Autodesk Inventor part; units mm, degrees
ref_plane "YZ Plane" through (0, 0, 0) normal (1, 0, 0) x (0, 1, 0)
ref_plane "XZ Plane" through (0, 0, 0) normal (0, 1, 0) x (-1, 0, 0)
ref_plane "XY Plane" through (0, 0, 0) normal (0, 0, 1) x (1, 0, 0)
sketch "Sketch1" plane through (0, 0, 0) normal (1, 0, 0) x (0, 1, 0)
  line L0 (0, 0) -> (-127, 0)
  line L1 (-127, 0) -> (-127, -127)
  line L2 (-127, -127) -> (0, -127)
  line L3 (0, -127) -> (0, -120.65)
  line L4 (0, -6.35) -> (0, 0)
  line L5 (0, -6.35) -> (-3.175, -6.35)
  line L6 (-3.175, -6.35) -> (-3.175, -3.175)
  line L7 (-3.175, -3.175) -> (-9.525, -3.175)
  line L8 (-9.525, -3.175) -> (-9.525, -6.35)
  line L9 (-3.175, -6.35) -> (0, -6.35)
  line L10 (0, -120.65) -> (-3.175, -120.65)
  line L11 (-3.175, -120.65) -> (-3.175, -123.825)
  line L12 (-3.175, -123.825) -> (-9.525, -123.825)
  line L13 (-9.525, -123.825) -> (-9.525, -120.65)
  line L14 (0, -120.65) -> (-3.175, -120.65)
  line L15 (-120.65, -6.35) -> (-120.65, -9.525)
  line L16 (-120.65, -9.525) -> (-123.825, -9.525)
  line L17 (-123.825, -9.525) -> (-123.825, -15.875)
  line L18 (-123.825, -15.875) -> (-120.65, -15.875)
  line L19 (-120.65, -9.525) -> (-120.65, -6.35)
  line L20 (-120.65, -120.65) -> (-120.65, -117.475)
  line L21 (-120.65, -117.475) -> (-123.825, -117.475)
  line L22 (-123.825, -117.475) -> (-123.825, -111.125)
  line L23 (-123.825, -111.125) -> (-120.65, -111.125)
  line L24 (-120.65, -120.65) -> (-120.65, -117.475)
  line L25 (-120.65, -111.125) -> (-120.65, -15.875)
  line L26 (-120.65, -6.35) -> (-107.95, -6.35)
  line L27 (-107.95, -6.35) -> (-107.95, -3.175)
  line L28 (-107.95, -3.175) -> (-101.6, -3.175)
  line L29 (-101.6, -3.175) -> (-101.6, -6.35)
  line L30 (-120.65, -6.35) -> (-107.95, -6.35)
  line L31 (-101.6, -6.35) -> (-9.525, -6.35)
  line L32 (-120.65, -120.65) -> (-107.95, -120.65)
  line L33 (-107.95, -120.65) -> (-107.95, -123.825)
  line L34 (-107.95, -123.825) -> (-101.6, -123.825)
  line L35 (-101.6, -123.825) -> (-101.6, -120.65)
  line L36 (-9.525, -120.65) -> (-101.6, -120.65)
  line L37 (-107.95, -120.65) -> (-120.65, -120.65)
  dimension "d0" = 127
  dimension "d1" = 127
  dimension "d2" = 6.35
  dimension "d3" = 120.65
  dimension "d4" = 114.3
  dimension "d5" = 3.175
  dimension "d9" = 3.175
  dimension "d10" = 3.175
  dimension "d11" = 3.175
  dimension "d12" = 6.35
  dimension "d13" = 3.175
  dimension "d14" = 3.175
  dimension "d15" = 6.35
  dimension "d16" = 3.175
  dimension "d17" = 3.175
  dimension "d18" = 6.35
  dimension "d21" = 12.7
  dimension "d22" = 3.175
  dimension "d23" = 6.35
  dimension "d24" = 12.7
  dimension "d25" = 3.175
  dimension "d26" = 6.35
extrude "Extrusion1" add sketch "Sketch1" along normal blind 304.8
properties part number "CompactSlidePart1" material "Aluminum 6061"
Verification items for the finished model (mm, model axes). A direction names the side the tool comes from. Coordinates: 2 decimals unless noted, no trailing zeros. Order: outer loops, then holes, each group sorted by start corner. A loop starts at its lowest first (then second) coordinate and runs counter-clockwise, first axis right, second up. Notation, with made-up numbers: M 34.5,17 L 52.5,17 A25 cw 52.5,52 Z; hole C 77,7 d4. An arc over 180 degrees is marked long. One line per item, written item: value. Start each with the question number.
Item 1: Sectioned sample at A-A on y = -113. Record the cut outline in (x, z), then the cut area to 3 significant figures.
Item 2: Sectioned sample at C-C on z = -23. Record the cut outline in (x, y), then the cut area to 3 significant figures.
Item 3: Mould release check, pull along Y, two halves, no side actions. Record for faces 4 (the flat face through (304.8, -125, -63)), 5 (the flat face through (150, -123.825, -13)), 6 (the flat face through (150, -105, -123.825)): pulls with the +Y half, pulls with the -Y half, needs draft (parallel to the pull), parting line crosses it, or undercut.
Item 4: Depth check by flat-ended pin: P1, Ø6, axis at x = 194.5, z = -53.5, coming from the +Y side. Enter the tip coordinate at first touch or a pass-through.
Item 5: Access from +Z, -Z, +X, -X, +Y, -Y to the whole of each face (thin tool, end or side, straight path). Record for faces 1 (the flat face through (150, -63, 0)), 2 (the flat face through (150, -114, -120.65)), 3 (the flat face through (150, -6, -3.175)).
Item 6: Thickness scan on probe 1 along Z at (x, y) = (150, -18); probe 2 along Y at (x, z) = (80, -71.5); probe 3 along Y at (x, z) = (72.5, -12) (3 decimals). Record the ranges inside material, lowest first.
Calculated:
1. outline: M 0,-127 L 304.8,-127 L 304.8,-120.65 L 0,-120.65 Z; M 0,-6.35 L 304.8,-6.35 L 304.8,0 L 0,0 Z
1. area: 3,870 mm^2
2. outline: M 0,-127 L 304.8,-127 L 304.8,-120.65 L 0,-120.65 Z
2. area: 1,940 mm^2
3. face 4: needs draft
3. face 5: pulls with the +Y half
3. face 6: undercut
4. P1: y = -120.65
5. face 1: +Z, +X, -X, +Y, -Y
5. face 2: +X, -X, +Y
5. face 3: +X, -X
6. probe 1: -127 to -120.65, -6.35 to 0
6. probe 2: -127 to -120.65
6. probe 3: -127 to -123.825
